from build123d import *

# Parameters (mm, degrees)
SKICA1_W                 = 120
SKICA1_H                 = 120
VYSUNOUT1_DEPTH          = 90
ZAOBLIT1_R               = 10
ZAOBLIT2_R               = 10
ZAOBLIT3_R               = 10
ZAOBLIT4_R               = 10
SKO_EPINA4_T             = -4
SKICA2_OUTSIDE_W         = 160.418
SKICA2_OUTSIDE_H         = 160.418
ODEBRAT_VYSUNUT_M1_DEPTH = 30


with BuildPart() as part:
    # Skica1 → Vysunout1 (new body)
    with BuildSketch(Plane.XY):
        with Locations((60, 60)):
            Rectangle(SKICA1_W, SKICA1_H)
    extrude(amount=VYSUNOUT1_DEPTH)

    # Zaoblit1
    zaoblit1_edges = [part.edges().sort_by_distance(p)[0] for p in [
        (120, 120, 45),
    ]]
    fillet(zaoblit1_edges, radius=ZAOBLIT1_R)

    # Zaoblit2
    zaoblit2_edges = [part.edges().sort_by_distance(p)[0] for p in [
        (0, 120, 45),
    ]]
    fillet(zaoblit2_edges, radius=ZAOBLIT2_R)

    # Zaoblit3
    zaoblit3_edges = [part.edges().sort_by_distance(p)[0] for p in [
        (0, 0, 45),
    ]]
    fillet(zaoblit3_edges, radius=ZAOBLIT3_R)

    # Zaoblit4
    zaoblit4_edges = [part.edges().sort_by_distance(p)[0] for p in [
        (120, 0, 45),
    ]]
    fillet(zaoblit4_edges, radius=ZAOBLIT4_R)

    # Skořepina4
    sko_epina4_openings = [part.faces().sort_by_distance(p)[0] for p in [
        (60, 60, 90),
    ]]
    offset(amount=SKO_EPINA4_T, openings=sko_epina4_openings, kind=Kind.INTERSECTION)

    # Skica2 outside → Odebrat vysunutím1 (cut)
    with BuildSketch(Plane.XY.offset(90)):
        with Locations((60, 60)):
            Rectangle(SKICA2_OUTSIDE_W, SKICA2_OUTSIDE_H)
        with BuildLine():
            Line((10, 2), (110, 2))
            ThreePointArc((110, 2), (115.656854249, 4.343145751), (118, 10))
            Line((118, 10), (118, 110))
            ThreePointArc((118, 110), (115.656854249, 115.656854249), (110, 118))
            Line((110, 118), (10, 118))
            ThreePointArc((10, 118), (4.343145751, 115.656854249), (2, 110))
            Line((2, 110), (2, 10))
            ThreePointArc((2, 10), (4.343145751, 4.343145751), (10, 2))
        make_face(mode=Mode.SUBTRACT)
    extrude(amount=-ODEBRAT_VYSUNUT_M1_DEPTH, mode=Mode.SUBTRACT)


solid = part.part
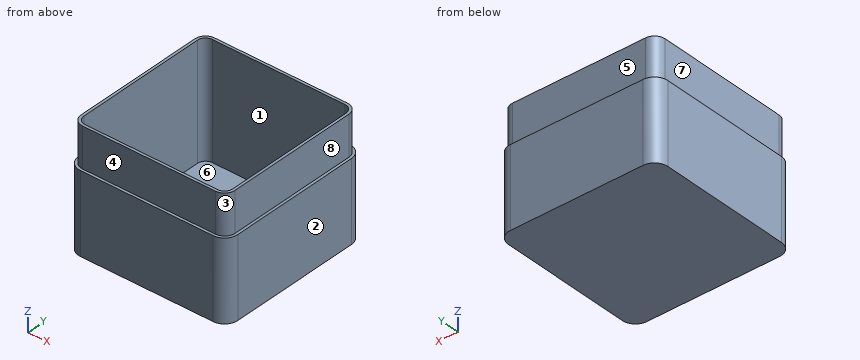
Build history of the part. All positions in model axes, mm. Face numbers are marked on the shaded views. A direction names the side the tool comes from. Coordinates: 2 decimals unless noted, no trailing zeros. Order: outer loops, then holes, each group sorted by start corner. A loop starts at its lowest first (then second) coordinate and runs counter-clockwise, first axis right, second up. Notation, with made-up numbers: (-37, 52) - (-14, 52) arc R19 ccw to (-14, 80) - close; hole circle Ø11 at (30, -39.5). An arc over 180 degrees is marked (long way). Write item = value, one per line. Start each with the question number.
1) Saw through at B-B on z = 11.5. Write the cut outline in (x, y).
2) Wall check: line 1 along X through (y, z) = (23.5, 11.5); line 2 along X through (y, z) = (56.5, 86). Give the ranges that are in metal, low to high. Write a range as from..to.
3) Flat gauge pins, fed straight in: pin 1 Ø24 at (x, z) = (47, 81) entering from -Y; pin 2 Ø24 at (x, z) = (61.5, 76.5) entering from +Y; pin 3 Ø2 at (x, y) = (52, 106) entering from -Z; pin 4 Ø15 at (y, z) = (40.5, 74) entering from +X. Where does each tip first touch, or does it go through?
4) 3-axis set-ups, long thin cutter, end or side, ignore diameter. For the marked faces 4, 5, 6, 7 and 8: which of +Z, -Z, +X, -X, +Y, -Y reach the whole face in a straight line?
5) Two-plate mould, pull along Y, no slides. Class the marked faces 1, 2 and 3: pulls with the +Y half, pulls with the -Y half, needs draft (parallel to the pull), parting line crosses it, or undercut.
6) Saw through at A-A on y = 83.5. Write the cut outline in (x, z).
From the geometry:
q1.outline = (0, 10) arc R10 ccw to (10, 0) - (110, 0) arc R10 ccw to (120, 10) - (120, 110) arc R10 ccw to (110, 120) - (10, 120) arc R10 ccw to (0, 110) - close; hole (4, 10) arc R6 ccw to (10, 4) - (110, 4) arc R6 ccw to (116, 10) - (116, 110) arc R6 ccw to (110, 116) - (10, 116) arc R6 ccw to (4, 110) - close
q2.line_1 = 0..4, 116..120
q2.line_2 = 2..4, 116..118
q3.pin_1 = 2
q3.pin_2 = 118
q3.pin_3 = 0
q3.pin_4 = 118
q4.face_4 = +Z, +X, -X, -Y
q4.face_5 = +Z, +X, -X, +Y
q4.face_6 = +Z
q4.face_7 = +Z, -X, +Y, -Y
q4.face_8 = +Z, +X, +Y, -Y
q5.face_1 = undercut
q5.face_2 = needs draft
q5.face_3 = pulls with the -Y half
q6.outline = (0, 0) - (120, 0) - (120, 60) - (118, 60) - (118, 90) - (116, 90) - (116, 4) - (4, 4) - (4, 90) - (2, 90) - (2, 60) - (0, 60) - close
